```python
from build123d import *

# Parameters (mm, degrees)
SKETCH1_W           = 4.3
SKETCH1_H           = 15
SKETCH1_W_2         = 50
SKETCH1_H_2         = 4
BOSS_EXTRUDE1_DEPTH = 4.3


with BuildPart() as part:
    # Sketch1 → Boss-Extrude1 (new body)
    with BuildSketch(Plane.XY):
        Polygon((0, 140), (11.393, 140), (11.393, 135.7), (26.393, 135.7), (26.393, 140), (37.836, 140), (37.836, 135.7), (52.836, 135.7), (52.836, 140), (64.279, 140), (64.279, 135.7), (79.279, 135.7), (79.279, 140), (90.722, 140), (90.722, 135.7), (105.722, 135.7), (105.722, 140), (117.165, 140), (117.165, 135.7), (132.165, 135.7), (132.165, 140), (143.608, 140), (143.608, 135.7), (158.608, 135.7), (158.608, 140), (170, 140), (170, 122.5), (165.7, 122.5), (165.7, 107.5), (170, 107.5), (170, 92.5), (165.7, 92.5), (165.7, 77.5), (170, 77.5), (170, 62.5), (165.7, 62.5), (165.7, 47.5), (170, 47.5), (170, 32.5), (165.7, 32.5), (165.7, 17.5), (170, 17.5), (170, 0), (158.758, 0), (158.758, -4.3), (143.458, -4.3), (143.458, 0), (132.315, 0), (132.315, -4.3), (117.015, -4.3), (117.015, 0), (105.872, 0), (105.872, -4.3), (90.572, -4.3), (90.572, 0), (79.429, 0), (79.429, -4.3), (64.129, -4.3), (64.129, 0), (52.986, 0), (52.986, -4.3), (37.686, -4.3), (37.686, 0), (26.543, 0), (26.543, -4.3), (11.243, -4.3), (11.243, 0), (0, 0), (0, 17.5), (4.3, 17.5), (4.3, 32.5), (0, 32.5), (0, 47.5), (4.3, 47.5), (4.3, 62.5), (0, 62.5), (0, 77.5), (4.3, 77.5), (4.3, 92.5), (0, 92.5), (0, 107.5), (4.3, 107.5), (4.3, 122.5), (0, 122.5), align=None)
        with Locations((69.45, 35)):
            Rectangle(SKETCH1_W, SKETCH1_H, mode=Mode.SUBTRACT)
        with Locations((69.45, 80)):
            Rectangle(SKETCH1_W, SKETCH1_H, mode=Mode.SUBTRACT)
        with Locations((49.15, 80)):
            Rectangle(SKETCH1_W, SKETCH1_H, mode=Mode.SUBTRACT)
        with Locations((85, 49.7)):
            Rectangle(SKETCH1_W_2, SKETCH1_H_2, mode=Mode.SUBTRACT)
        with Locations((85, 93.7)):
            Rectangle(SKETCH1_W_2, SKETCH1_H_2, mode=Mode.SUBTRACT)
        with BuildLine():
            Line((53.173708042, 114.65), (65.426291958, 114.65))
            ThreePointArc((65.426291958, 114.65), (66.75120362, 115.19879638), (67.3, 116.523708042))
            Line((67.3, 116.523708042), (67.3, 120.776291958))
            ThreePointArc((67.3, 120.776291958), (66.75120362, 122.10120362), (65.426291958, 122.65))
            Line((65.426291958, 122.65), (53.173708042, 122.65))
            ThreePointArc((53.173708042, 122.65), (51.84879638, 122.10120362), (51.3, 120.776291958))
            Line((51.3, 120.776291958), (51.3, 116.523708042))
            ThreePointArc((51.3, 116.523708042), (51.84879638, 115.19879638), (53.173708042, 114.65))
        make_face(mode=Mode.SUBTRACT)
        with BuildLine():
            Line((53.173708042, 98.65), (65.426291958, 98.65))
            ThreePointArc((65.426291958, 98.65), (66.75120362, 99.19879638), (67.3, 100.523708042))
            Line((67.3, 100.523708042), (67.3, 104.776291958))
            ThreePointArc((67.3, 104.776291958), (66.75120362, 106.10120362), (65.426291958, 106.65))
            Line((65.426291958, 106.65), (53.173708042, 106.65))
            ThreePointArc((53.173708042, 106.65), (51.84879638, 106.10120362), (51.3, 104.776291958))
            Line((51.3, 104.776291958), (51.3, 100.523708042))
            ThreePointArc((51.3, 100.523708042), (51.84879638, 99.19879638), (53.173708042, 98.65))
        make_face(mode=Mode.SUBTRACT)
        with Locations((49.15, 35)):
            Rectangle(SKETCH1_W, SKETCH1_H, mode=Mode.SUBTRACT)
        with BuildLine():
            Line((56.3, 9), (62.3, 9))
            ThreePointArc((62.3, 9), (63.714213562, 9.585786438), (64.3, 11))
            Line((64.3, 11), (64.3, 17))
            ThreePointArc((64.3, 17), (63.714213562, 18.414213562), (62.3, 19))
            Line((62.3, 19), (56.3, 19))
            ThreePointArc((56.3, 19), (54.885786438, 18.414213562), (54.3, 17))
            Line((54.3, 17), (54.3, 11))
            ThreePointArc((54.3, 11), (54.885786438, 9.585786438), (56.3, 9))
        make_face(mode=Mode.SUBTRACT)
        with BuildLine():
            Line((56.3, 65.7), (62.3, 65.7))
            ThreePointArc((62.3, 65.7), (63.714213562, 65.114213562), (64.3, 63.7))
            Line((64.3, 63.7), (64.3, 57.7))
            ThreePointArc((64.3, 57.7), (63.714213562, 56.285786438), (62.3, 55.7))
            Line((62.3, 55.7), (56.3, 55.7))
            ThreePointArc((56.3, 55.7), (54.885786438, 56.285786438), (54.3, 57.7))
            Line((54.3, 57.7), (54.3, 63.7))
            ThreePointArc((54.3, 63.7), (54.885786438, 65.114213562), (56.3, 65.7))
        make_face(mode=Mode.SUBTRACT)
    extrude(amount=BOSS_EXTRUDE1_DEPTH)


solid = part.part
```
Can you work these out from the model? Positions are in its coordinate system, mm. A direction names the side the tool comes from. Coordinates: 2 decimals unless noted, no trailing zeros. Order: outer loops, then holes, each group sorted by start corner. A loop starts at its lowest first (then second) coordinate and runs counter-clockwise, first axis right, second up. Notation, with made-up numbers: (72.25, 61) - (118.25, 61) arc R13 cw to (118.25, 82) - close; hole circle Ø1 at (30, -25). An arc over 180 degrees is marked (long way). Answer in a Markdown table with one row per item.
1. Suppose I cut it at C-C (z = 2.1). Give the number of separate pieces and of enclosed holes in the cut face, and give its area (3 significant figures).
Reply:
| item | result |
|---|---|
| separate pieces | 1 |
| enclosed holes | 10 |
| area | 22,200 mm^2 |
2. Suppose I cut it at B-B (x = 103). Please give me the cut outline in (y, z).
Reply:
| item | result |
|---|---|
| outline | (-4.3, 0) - (47.7, 0) - (47.7, 4.3) - (-4.3, 4.3) - close; (51.7, 0) - (91.7, 0) - (91.7, 4.3) - (51.7, 4.3) - close; (95.7, 0) - (135.7, 0) - (135.7, 4.3) - (95.7, 4.3) - close |
3. For faces 4 (the flat face through (59, 98.65, 2)), 5 (the flat face through (32, 0, 2)), 6 (the flat face through (151, 135.7, 2)), which set-ups out of +Z, -Z, +X, -X, +Y, -Y let a thin tool reach every point of the face, with its end or its side?
Reply:
| item | result |
|---|---|
| face 4 | +Z, -Z |
| face 5 | +Z, -Z, -Y |
| face 6 | +Z, -Z, +Y |
4. Suppose I cut it at A-A (y = 37.5). Please give me the cut outline in (x, z), and give its area (3 significant figures).
Reply:
| item | result |
|---|---|
| outline | (0, 0) - (47, 0) - (47, 4.3) - (0, 4.3) - close; (51.3, 0) - (67.3, 0) - (67.3, 4.3) - (51.3, 4.3) - close; (71.6, 0) - (170, 0) - (170, 4.3) - (71.6, 4.3) - close |
| area | 694 mm^2 |
5. If I drill on line 1 along Y through (x, z) = (80, 2.55); line 2 along X through (y, z) = (40.5, 1.6); line 3 along Y through (x, z) = (103, 3.95), over which ranges is the centre line in solid material (lowest first)?
Reply:
| item | result |
|---|---|
| line 1 | y = 0 to 47.7, 51.7 to 91.7, 95.7 to 140 |
| line 2 | x = 0 to 47, 51.3 to 67.3, 71.6 to 170 |
| line 3 | y = -4.3 to 47.7, 51.7 to 91.7, 95.7 to 135.7 |
6. For pin 1 (2 mm diameter, centred on x = 7.5, z = 2, fed in from -Y); pin 2 (2 mm diameter, centred on x = 101.5, z = 2.5, fed in from +Y); pin 3 (1.3 mm diameter, centred on y = 25.5, z = 2, fed in from +X), each with a flat end and sliding along its axis, tell me the tip position at first contact or that it passes through.
Reply:
| item | result |
|---|---|
| pin 1 | stops at y = 0 |
| pin 2 | stops at y = 135.7 |
| pin 3 | stops at x = 165.7 |
7. If we mould it in two halves opening along X, with no side actions, what happens to faces 1 (the flat face through (79.429, -2, 2)), 2 (the flat face through (151, -4.3, 2)), 3 (the flat face through (4.3, 25, 2))? For each: pulls with the +X half, pulls with the -X half, needs draft (parallel to the pull), parting line crosses it, or undercut.
Reply:
| item | result |
|---|---|
| face 1 | undercut |
| face 2 | needs draft |
| face 3 | pulls with the -X half |
8. Suppose I cut it at D-D (y = 22.5). Please give me the cut outline in (x, z).
Reply:
| item | result |
|---|---|
| outline | (4.3, 0) - (165.7, 0) - (165.7, 4.3) - (4.3, 4.3) - close |
